Could you check a few things on this model? Use its own coordinates, in mm. Face numbers are marked on the shaded views. A direction names the side the tool comes from. Give positions to 0.01 mm unless a question says otherwise; leave off trailing zeros. Loops run counter-clockwise (first coordinate to the right, second up) from the corner with the lowest first, then second, coordinate; pieces in that order, holes last. Notation, with made-up numbers: (69, 25.25) - (109, 25.25) arc R16 cw to (109, 46.25) - close; hole circle Ø5 at (45, -35.75). An arc over 180 degrees is marked (long way). Write each question's results on one line, items separated by ' | '. Start each with the question number.
1) I want a section at C-C, the plane z = -9. Write out the boundary of the cut face in (x, y).
2) If we mould it in two halves opening along Y, with no side actions, what happens to the marked faces 1, 2 and 3? For each: +Y half, -Y half, draft (parallel to the pull), parting line (faces both ways), or undercut.
3) If I drill on probe 1 along X at (y, z) = (0, -4); probe 2 along Z at (x, y) = (35, 0), over which ranges is the centre line in solid material (lowest first)? Write a range as [from, to].
4) On a 3-axis mill with a long thin cutter (end or side, diameter ignored), from which of +Z, -Z, +X, -X, +Y, -Y can I reach the whole of each face in a straight line? I mean the marked faces 4, 5 and 6. Say none if no direction works.
5) I'm going to push flat-ended pins straight in: pin 1 (3 mm diameter, centred on x = 16.5, y = -12.5, fed in from -Z); pin 2 (12 mm diameter, centred on x = -8, y = -12, fed in from -Z); pin 3 (3 mm diameter, centred on y = -2, z = -40.5, fed in from +X). Where does each tip first touch, or does it pass through?
6) I want a section at D-D, the plane y = -8. Write out the boundary of the cut face in (x, z).
7) I want a section at B-B, the plane x = 32. Write out the boundary of the cut face in (y, z), and give its area (3 significant figures).
8) I want a section at A-A, the plane y = 0. Write out the boundary of the cut face in (x, z).
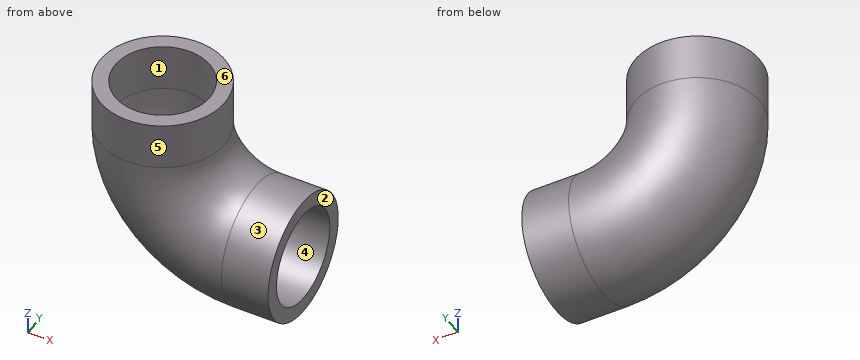
from build123d import *

# Parameters (mm, degrees)
SKETCH1_R   = 16.7005
SKETCH1_R_2 = 12.7


with BuildPart() as part:
    # Sweep1: sweep along a path in Sketch2
    with BuildLine(Plane(origin=(0, 0, 0), x_dir=(1, 0, 0), z_dir=(0, 1, 0))) as sweep1_path:
        Line((0, 0), (0, 12.7))
        ThreePointArc((0, 12.7), (7.439487758, 30.660512242), (25.4, 38.1))
        Line((25.4, 38.1), (38.1, 38.1))
    # Sketch1 → Sweep1 (sweep)
    with BuildSketch(Plane.XY):
        Circle(SKETCH1_R)
        Circle(SKETCH1_R_2, mode=Mode.SUBTRACT)
    sweep(path=sweep1_path.line)


solid = part.part
Answers:
1) outline: circle Ø33.4 at (0, 0); hole circle Ø25.4 at (0, 0)
2) face 1: undercut | face 2: draft | face 3: parting line
3) probe 1: x = [-16.7, -12.7], [12.7, 16.7] | probe 2: z = [-54.8, -50.8], [-25.4, -21.4]
4) face 4: +X | face 5: +Z | face 6: +Z, +X, -X, +Y, -Y
5) pin 1: stops at z = -49.65 | pin 2: stops at z = -40.43 | pin 3: stops at x = 1.34
6) outline: (-14.66, -12.7) arc R40.06 ccw to (25.4, -52.76) - (38.1, -52.76) - (38.1, -47.96) - (25.4, -47.96) arc R35.26 cw to (-9.86, -12.7) - (-9.86, 0) - (-14.66, 0) - close; (9.86, -12.7) arc R15.54 ccw to (25.4, -28.24) - (38.1, -28.24) - (38.1, -23.44) - (25.4, -23.44) arc R10.74 cw to (14.66, -12.7) - (14.66, 0) - (9.86, 0) - close
7) outline: circle Ø33.4 at (0, -38.1); hole circle Ø25.4 at (0, -38.1) | area: 370 mm2
8) outline: (-16.7, -12.7) arc R42.1 ccw to (25.4, -54.8) - (38.1, -54.8) - (38.1, -50.8) - (25.4, -50.8) arc R38.1 cw to (-12.7, -12.7) - (-12.7, 0) - (-16.7, 0) - close; (12.7, -12.7) arc R12.7 ccw to (25.4, -25.4) - (38.1, -25.4) - (38.1, -21.4) - (25.4, -21.4) arc R8.7 cw to (16.7, -12.7) - (16.7, 0) - (12.7, 0) - close
